```python
from build123d import *

# Parameters (mm, degrees)
BOSS_EXTRUDE1_DEPTH   = 6.6
CUT_EXTRUDE1_DEPTH    = 2.4
F_3_0MM_DOWEL_HOLE1_D = 3


with BuildPart() as part:
    # Sketch1 → Boss-Extrude1 (new body)
    with BuildSketch(Plane(origin=(0, 0, 0), x_dir=(1, 0, 0), z_dir=(0, 1, 0))):
        Polygon((-5.875, 3.391932831), (-5.875, -3.391932831), (0, -6.783865663), (5.875, -3.391932831), (5.875, 3.391932831), (0, 6.783865663), align=None)
    extrude(amount=BOSS_EXTRUDE1_DEPTH)

    # Sketch2 → Cut-Extrude1 (cut)
    with BuildSketch(Plane(origin=(0, 6.6, 0), x_dir=(1, 0, 0), z_dir=(0, 1, 0))):
        with BuildLine():
            Line((-3.125, 2.75), (-3.125, -2.75))
            ThreePointArc((-3.125, -2.75), (0, -4.316681548), (3.125, -2.75))
            Line((3.125, -2.75), (3.125, 2.75))
            ThreePointArc((3.125, 2.75), (0, 4.316681548), (-3.125, 2.75))
        make_face()
    extrude(amount=-CUT_EXTRUDE1_DEPTH, mode=Mode.SUBTRACT)

    # Ø3.0mm Dowel Hole1 (through all)
    with Locations(Plane(origin=(0, 0, 0), x_dir=(-1, 0, 0), z_dir=(0, -1, 0))):
        with Locations((0, 0)):
            Hole(F_3_0MM_DOWEL_HOLE1_D / 2)


solid = part.part
```
Source: CAD feature listing. Evaluate the final solid. Frame: model axes, mm. A direction names the side the tool comes from. Give positions to 0.01 mm unless a question says otherwise; leave off trailing zeros. Loops run counter-clockwise (first coordinate to the right, second up) from the corner with the lowest first, then second, coordinate; pieces in that order, holes last. Notation, with made-up numbers: (-19.75, 18) -> (-14.75, 18) arc R18 cw to (-14.75, 53) -> close; hole circle Ø6 at (52, 56). An arc over 180 degrees is marked (long way). Use a Markdown table: item, result. Add a question column.
(1) Section query D-D (x = -2.75). Output: boundary loops of the cut face in (y, z), then the cut area to 3 significant figures.
(2) Section query B-B (y = 1). Output: boundary loops of the cut face in (x, z) (3 decimals), then the cut area to 3 significant figures.
(3) First-contact query: pin 1 Ø3 at (x, z) = (-1.5, 0) entering from +Y. Flat tip, straight axial feed; report the tip coordinate or a pass-through.
(4) Ray query, line 1 (Y direction, x = -0.25, z = 3.25); line 2 (X direction, y = 2, z = 0.75) (3 decimals); line 3 (X direction, y = 5.25, z = 3.25) (3 decimals). Return the intervals inside material, ascending.
(5) Access query for faces 1 (the face through (-4, 6.6, 0)), 2 (the face through (3.125, 5, 0)). Directions: +Z, -Z, +X, -X, +Y, -Y. A direction counts if a zero-diameter tool reaches every point of the face in a straight line with its end or side. Return the directions, or none.
(6) Pull-direction query (X, two-part tool) for faces 3 (the face through (-1.4, 0, 1.4)), 4 (the face through (2.9, 3.25, 5.11)), 5 (the face through (-1.4, 4.2, 0.9)); classes: +X half, -X half, draft (parallel to the pull), parting line (faces both ways), or undercut.
(7) Section query A-A (z = 0). Output: boundary loops of the cut face in (x, y) (3 decimals).
(8) Section query C-C (z = -2.5). Output: boundary loops of the cut face in (x, y) (3 decimals).
Checked values:
| question | item | result |
|---|---|---|
| 1 | outline | (0, -5.2) -> (6.6, -5.2) -> (6.6, -3.18) -> (4.2, -3.18) -> (4.2, 3.18) -> (6.6, 3.18) -> (6.6, 5.2) -> (0, 5.2) -> close |
| 1 | area | 53.3 mm^2 |
| 2 | outline | (-5.875, -3.392) -> (0, -6.784) -> (5.875, -3.392) -> (5.875, 3.392) -> (0, 6.784) -> (-5.875, 3.392) -> close; hole circle Ø3 at (0, 0) |
| 2 | area | 112 mm^2 |
| 3 | pin 1 | y = 4.2 |
| 4 | line 1 | 0 to 4.2 |
| 4 | line 2 | -5.875 to -1.299, 1.299 to 5.875 |
| 4 | line 3 | -5.875 to -2.68, 2.68 to 5.875 |
| 5 | face 1 | +Z, -Z, +X, -X, +Y |
| 5 | face 2 | +Y |
| 6 | face 3 | draft |
| 6 | face 4 | +X half |
| 6 | face 5 | undercut |
| 7 | outline | (-5.875, 0) -> (-1.5, 0) -> (-1.5, 4.2) -> (-3.125, 4.2) -> (-3.125, 6.6) -> (-5.875, 6.6) -> close; (1.5, 0) -> (5.875, 0) -> (5.875, 6.6) -> (3.125, 6.6) -> (3.125, 4.2) -> (1.5, 4.2) -> close |
| 8 | outline | (-5.875, 0) -> (5.875, 0) -> (5.875, 6.6) -> (3.125, 6.6) -> (3.125, 4.2) -> (-3.125, 4.2) -> (-3.125, 6.6) -> (-5.875, 6.6) -> close |
